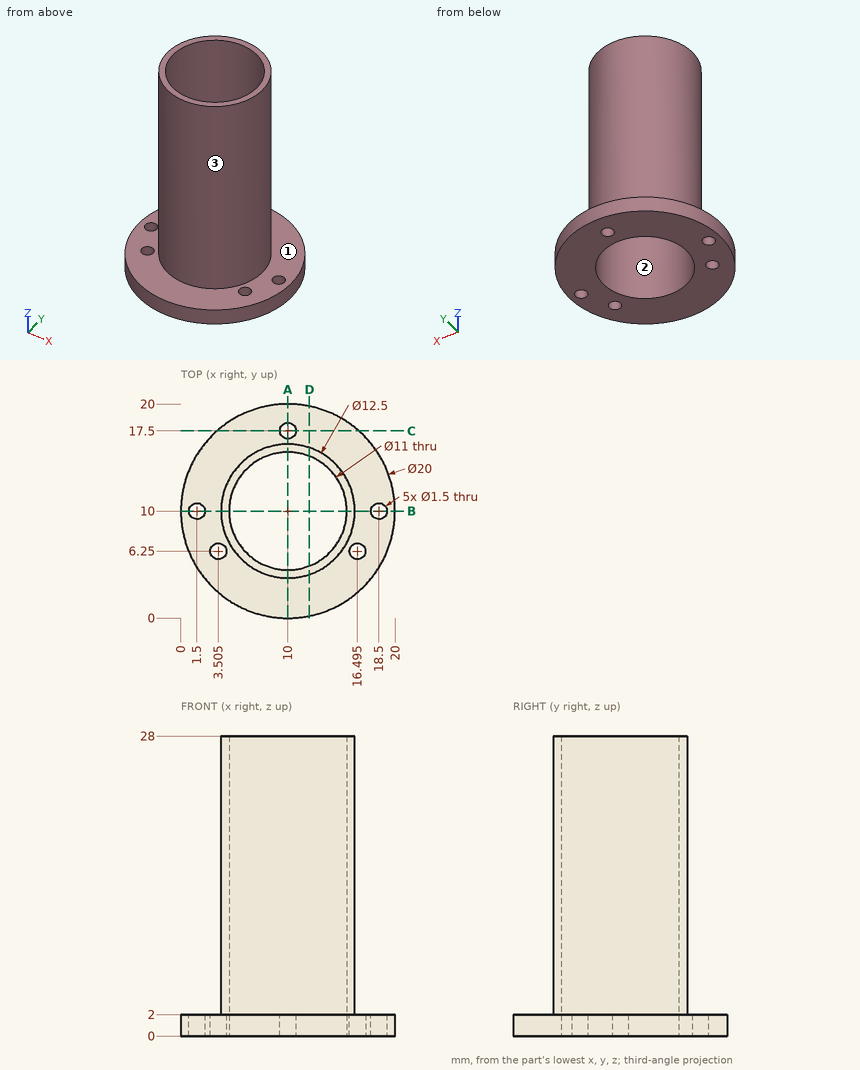
Drawing for the job (mm, zero at the part's lowest x, y, z). Give positions to 0.01 mm unless a question says otherwise; leave off trailing zeros. Loops run counter-clockwise (first coordinate to the right, second up) from the corner with the lowest first, then second, coordinate; pieces in that order, holes last. Notation, with made-up numbers: M -5.5,23 L 34.5,23 A23 ccw 34.5,45 Z; hole C 84.25,-0.5 d7. An arc over 180 degrees is marked long. One line per question, with ' | ' between items. Start each with the question number.
1. Flat gauge pins, fed straight in: pin 1 (2 mm diameter, centred on x = 18.5, y = 10, fed in from +Z); pin 2 (6 mm diameter, centred on x = 10.5, z = 16.5, fed in from +Y); pin 3 (10 mm diameter, centred on y = 4.5, z = 21.5, fed in from -X). Where does each tip first touch, or does it go through?
2. Saw through at B-B on y = 10. Give the cut face in (x, z).
3. Two-plate mould, pull along X, no slides. Class the marked faces 1, 2 and 3: pulls with the +X half, pulls with the -X half, needs draft (parallel to the pull), parting line crosses it, or undercut.
4. Saw through at C-C on y = 17.5. Give the cut face in (x, z).
5. Saw through at A-A on x = 10. Give the cut face in (y, z).
6. Saw through at D-D on x = 12. Give the cut face in (y, z).
7. Probe L1, parallel to Y at x = 10, z = 0.6; L2, parallel to Y at x = 10, z = 20.5; L3, parallel to Y at x = 1.5, z = 0.8. List the from-to ranges inside material, lowest first. Write a range as from..to.
Result sheet:
1) pin 1: stops at z = 2 | pin 2: stops at y = 16.25 | pin 3: stops at x = 3.77
2) outline: M 0,0 L 0.75,0 L 0.75,2 L 0,2 Z; M 2.25,0 L 4.5,0 L 4.5,28 L 3.75,28 L 3.75,2 L 2.25,2 Z; M 15.5,0 L 17.75,0 L 17.75,2 L 16.25,2 L 16.25,28 L 15.5,28 Z; M 19.25,0 L 20,0 L 20,2 L 19.25,2 Z
3) face 1: needs draft | face 2: undercut | face 3: parting line crosses it
4) outline: M 3.39,0 L 9.25,0 L 9.25,2 L 3.39,2 Z; M 10.75,0 L 16.61,0 L 16.61,2 L 10.75,2 Z
5) outline: M 0,0 L 4.5,0 L 4.5,28 L 3.75,28 L 3.75,2 L 0,2 Z; M 15.5,0 L 16.75,0 L 16.75,2 L 16.25,2 L 16.25,28 L 15.5,28 Z; M 18.25,0 L 20,0 L 20,2 L 18.25,2 Z
6) outline: M 0.2,0 L 4.88,0 L 4.88,28 L 4.08,28 L 4.08,2 L 0.2,2 Z; M 15.12,0 L 19.8,0 L 19.8,2 L 15.92,2 L 15.92,28 L 15.12,28 Z
7) L1: y = 0..4.5, 15.5..16.75, 18.25..20 | L2: y = 3.75..4.5, 15.5..16.25 | L3: y = 4.73..9.25, 10.75..15.27
